Verification items for the finished model (mm, model axes). A direction names the side the tool comes from. Coordinates: 2 decimals unless noted, no trailing zeros. Order: outer loops, then holes, each group sorted by start corner. A loop starts at its lowest first (then second) coordinate and runs counter-clockwise, first axis right, second up. Notation, with made-up numbers: M -17,70.25 L 20,70.25 A7 cw 20,80.25 Z; hole C -27.5,81 d7. An arc over 180 degrees is marked long. Answer as a JSON object with one key per item and string values. Group by question number.
(1) Cross-section at D-D (x = 380). Enter the section's corners in (y, z).
(2) Material ranges on line 1 (Z direction, x = -173, y = -43.5); line 2 (Y direction, x = -300, z = -55); line 3 (Y direction, x = -3.5, z = -35.5), recorded low to high.
(3) Cross-section at B-B (x = -87). Enter the section's corners in (y, z).
(4) Mould release check, pull along X, two halves, no side actions. Record for faces 5 (the face through (-400, 22, 9)), 6 (the face through (310, 245, -55)), 7 (the face through (-220, 232, 10)): released by +X, released by -X, zero draft, split by the parting line, or undercut.
(5) Cross-section at A-A (x = -300). Enter the section's corners in (y, z).
(6) Gauge pin test, flat ends, axial feed: pin 1 Ø23 at (x, y) = (-220, 245) entering from +Z; pin 2 Ø3 at (x, z) = (309.5, 22.5) entering from +Y; pin 3 Ø3 at (x, z) = (284.5, -28.5) entering from +Y; pin 4 Ø18 at (x, y) = (-300, 245) entering from +Z. Record the tip position at first contact, or that the pin passes through.
(7) Cross-section at C-C (z = -73). Enter the section's corners in (x, y), plus the area to 3 significant figures.
(8) Access from +Z, -Z, +X, -X, +Y, -Y to the whole of each face (thin tool, end or side, straight path). Record for faces 1 (the face through (-391.445, -215.979, -27.03)), 2 (the face through (389, 238, -60)), 3 (the face through (-391.445, 215.979, 65.77)), 4 (the face through (300, 232, 10)).
from build123d import *

# Parameters (mm, degrees)
SKETCH_1_W      = 800
SKETCH_1_H      = 450
EXTRUDE_1_DEPTH = 150
SKETCH_2_R      = 10
EXTRUDE_2_DEPTH = 10
SKETCH_3_W      = 800
SKETCH_3_H      = 130
EXTRUDE_3_DEPTH = 50
SKETCH_4_W      = 800
SKETCH_4_H      = 450
EXTRUDE_4_DEPTH = 150
EXTRUDE_START   = -10
SKETCH_5_R      = 10
EXTRUDE_5_DEPTH = 10
FILLET_1_R      = 30


with BuildPart() as part:
    # 草图1 → 凸台-拉伸1 (new body)
    with BuildSketch(Plane.XY):
        Rectangle(SKETCH_1_W, SKETCH_1_H)
    extrude(amount=EXTRUDE_1_DEPTH)

    # 草图2 → 凸台-拉伸2 (add)
    # profile 1 of 6: a face of its own
    with BuildSketch(Plane(origin=(0, 0, 0), x_dir=(-1, 0, 0), z_dir=(0, 0, -1))):
        with BuildLine():
            Line((400, 245), (400, 225))
            Line((400, 225), (360, 225))
            Line((360, 225), (360, 245))
            ThreePointArc((360, 245), (380, 265), (400, 245))
        make_face()
        with Locations((380, 245)):
            Circle(SKETCH_2_R, mode=Mode.SUBTRACT)
    # profile 2 of 6: a face of its own
    with BuildSketch(Plane(origin=(0, 0, 0), x_dir=(-1, 0, 0), z_dir=(0, 0, -1))):
        with BuildLine():
            Line((240, 245), (240, 225))
            Line((240, 225), (200, 225))
            Line((200, 225), (200, 245))
            ThreePointArc((200, 245), (220, 265), (240, 245))
        make_face()
        with Locations((220, 245)):
            Circle(SKETCH_2_R, mode=Mode.SUBTRACT)
    # profile 3 of 6: a face of its own
    with BuildSketch(Plane(origin=(0, 0, 0), x_dir=(-1, 0, 0), z_dir=(0, 0, -1))):
        with BuildLine():
            Line((-200, 245), (-200, 225))
            Line((-200, 225), (-240, 225))
            Line((-240, 225), (-240, 245))
            ThreePointArc((-240, 245), (-220, 265), (-200, 245))
        make_face()
        with Locations((-220, 245)):
            Circle(SKETCH_2_R, mode=Mode.SUBTRACT)
    # profile 4 of 6: a face of its own
    with BuildSketch(Plane(origin=(0, 0, 0), x_dir=(-1, 0, 0), z_dir=(0, 0, -1))):
        with BuildLine():
            Line((-360, 245), (-360, 225))
            Line((-360, 225), (-400, 225))
            Line((-400, 225), (-400, 245))
            ThreePointArc((-400, 245), (-380, 265), (-360, 245))
        make_face()
        with Locations((-380, 245)):
            Circle(SKETCH_2_R, mode=Mode.SUBTRACT)
    # profile 5 of 6: a face of its own
    with BuildSketch(Plane(origin=(0, 0, 0), x_dir=(-1, 0, 0), z_dir=(0, 0, -1))):
        with BuildLine():
            Line((-280, 245), (-280, 225))
            Line((-280, 225), (-320, 225))
            Line((-320, 225), (-320, 245))
            ThreePointArc((-320, 245), (-300, 265), (-280, 245))
        make_face()
        with Locations((-300, 245)):
            Circle(SKETCH_2_R, mode=Mode.SUBTRACT)
    # profile 6 of 6: a face of its own
    with BuildSketch(Plane(origin=(0, 0, 0), x_dir=(-1, 0, 0), z_dir=(0, 0, -1))):
        with BuildLine():
            Line((320, 245), (320, 225))
            Line((320, 225), (280, 225))
            Line((280, 225), (280, 245))
            ThreePointArc((280, 245), (300, 265), (320, 245))
        make_face()
        with Locations((300, 245)):
            Circle(SKETCH_2_R, mode=Mode.SUBTRACT)
    extrude(amount=-EXTRUDE_2_DEPTH)

    # 草图3 → 凸台-拉伸3 (add)
    with BuildSketch(Plane(origin=(0, 0, 0), x_dir=(-1, 0, 0), z_dir=(0, 0, -1))):
        with BuildLine():
            Line((-40, 225), (40, 225))
            ThreePointArc((40, 225), (60, 205), (40, 185))
            Line((40, 185), (-40, 185))
            ThreePointArc((-40, 185), (-60, 205), (-40, 225))
        make_face()
        with Locations((0, -160)):
            Rectangle(SKETCH_3_W, SKETCH_3_H)
    extrude(amount=EXTRUDE_3_DEPTH)

    # 草图4 → 凸台-拉伸4 (add)
    with BuildSketch(Plane(origin=(0, 0, -50), x_dir=(-1, 0, 0), z_dir=(0, 0, -1))):
        Rectangle(SKETCH_4_W, SKETCH_4_H)
    extrude(amount=EXTRUDE_4_DEPTH)

    # 草图5 → 凸台-拉伸5 (add)
    # profile 1 of 6: a face of its own
    with BuildSketch(Plane.XY.offset(-50).offset(EXTRUDE_START)):
        with BuildLine():
            Line((400, 245), (400, 225))
            Line((400, 225), (360, 225))
            Line((360, 225), (360, 245))
            ThreePointArc((360, 245), (380, 265), (400, 245))
        make_face()
        with Locations(Location((380, 245, 0), (0, 0, 180))):
            Circle(SKETCH_5_R, mode=Mode.SUBTRACT)
    # profile 2 of 6: a face of its own
    with BuildSketch(Plane.XY.offset(-50).offset(EXTRUDE_START)):
        with BuildLine():
            Line((240, 245), (240, 225))
            Line((240, 225), (200, 225))
            Line((200, 225), (200, 245))
            ThreePointArc((200, 245), (220, 265), (240, 245))
        make_face()
        with Locations(Location((220, 245, 0), (0, 0, 180))):
            Circle(SKETCH_5_R, mode=Mode.SUBTRACT)
    # profile 3 of 6: a face of its own
    with BuildSketch(Plane.XY.offset(-50).offset(EXTRUDE_START)):
        with BuildLine():
            Line((-200, 245), (-200, 225))
            Line((-200, 225), (-240, 225))
            Line((-240, 225), (-240, 245))
            ThreePointArc((-240, 245), (-220, 265), (-200, 245))
        make_face()
        with Locations(Location((-220, 245, 0), (0, 0, 180))):
            Circle(SKETCH_5_R, mode=Mode.SUBTRACT)
    # profile 4 of 6: a face of its own
    with BuildSketch(Plane.XY.offset(-50).offset(EXTRUDE_START)):
        with BuildLine():
            Line((-360, 245), (-360, 225))
            Line((-360, 225), (-400, 225))
            Line((-400, 225), (-400, 245))
            ThreePointArc((-400, 245), (-380, 265), (-360, 245))
        make_face()
        with Locations(Location((-380, 245, 0), (0, 0, 180))):
            Circle(SKETCH_5_R, mode=Mode.SUBTRACT)
    # profile 5 of 6: a face of its own
    with BuildSketch(Plane.XY.offset(-50).offset(EXTRUDE_START)):
        with BuildLine():
            Line((-280, 245), (-280, 225))
            Line((-280, 225), (-320, 225))
            Line((-320, 225), (-320, 245))
            ThreePointArc((-320, 245), (-300, 265), (-280, 245))
        make_face()
        with Locations(Location((-300, 245, 0), (0, 0, 180))):
            Circle(SKETCH_5_R, mode=Mode.SUBTRACT)
    # profile 6 of 6: a face of its own
    with BuildSketch(Plane.XY.offset(-50).offset(EXTRUDE_START)):
        with BuildLine():
            Line((320, 245), (320, 225))
            Line((320, 225), (280, 225))
            Line((280, 225), (280, 245))
            ThreePointArc((280, 245), (300, 265), (320, 245))
        make_face()
        with Locations(Location((300, 245, 0), (0, 0, 180))):
            Circle(SKETCH_5_R, mode=Mode.SUBTRACT)
    extrude(amount=EXTRUDE_5_DEPTH)

    # 圆角1
    fillet_1_edges = [part.edges().sort_by_distance(p)[0] for p in [
        (0, 225, -200),
        (-400, 225, -130),
        (400, 0, -200),
        (400, 225, -130),
        (0, -225, -200),
        (-400, 0, -200),
        (-400, 0, 150),
        (0, -225, 150),
        (400, 0, 150),
        (400, -225, -25),
        (-400, -225, -25),
        (-400, 225, 80),
        (400, 225, 80),
        (0, 225, 150),
    ]]
    fillet(fillet_1_edges, radius=FILLET_1_R)


solid = part.part
Taken from the geometry:
{
 "1": {"outline": "M -223.28,-170 A28.28 ccw -195,-198.28 L 195,-198.28 A28.28 ccw 223.28,-170 L 223.28,-60 L 235,-60 L 235,-50 L -95,-50 L -95,0 L 235,0 L 235,10 L 223.28,10 L 223.28,120 A28.28 ccw 195,148.28 L -195,148.28 A28.28 ccw -223.28,120 Z; M 255,-60 L 265,-60 L 265,-50 L 255,-50 Z; M 255,0 L 265,0 L 265,10 L 255,10 Z"},
 "2": {"line 1": "z = -200 to -50, 0 to 150", "line 2": "y = -225 to 235, 255 to 265", "line 3": "y = -225 to -95, 185 to 225"},
 "3": {"outline": "M -225,-170 A30 ccw -195,-200 L 195,-200 A30 ccw 225,-170 L 225,-50 L -95,-50 L -95,0 L 225,0 L 225,120 A30 ccw 195,150 L -195,150 A30 ccw -225,120 Z"},
 "4": {"face 5": "released by -X", "face 6": "undercut", "face 7": "zero draft"},
 "5": {"outline": "M -225,-170 A30 ccw -195,-200 L 195,-200 A30 ccw 225,-170 L 225,-60 L 235,-60 L 235,-50 L -95,-50 L -95,0 L 235,0 L 235,10 L 225,10 L 225,120 A30 ccw 195,150 L -195,150 A30 ccw -225,120 Z; M 255,-60 L 265,-60 L 265,-50 L 255,-50 Z; M 255,0 L 265,0 L 265,10 L 255,10 Z"},
 "6": {"pin 1": "stops at z = 10", "pin 2": "stops at y = 225", "pin 3": "stops at y = -95", "pin 4": "passes through"},
 "7": {"outline": "M -400,-195 A30 ccw -370,-225 L 370,-225 A30 ccw 400,-195 L 400,195 A30 ccw 370,225 L -370,225 A30 ccw -400,195 Z", "area": "359,000 mm²"},
 "8": {"face 1": "+Z, -Z, -X, -Y", "face 2": "-Z, +X, +Y", "face 3": "+Z, -X, +Y", "face 4": "+Z, +X, -X, +Y"}
}
